Build history of the part. All positions in model axes, mm. A direction names the side the tool comes from. Coordinates: 2 decimals unless noted, no trailing zeros. Loops run counter-clockwise (first coordinate to the right, second up) from the corner with the lowest first, then second, coordinate; pieces in that order, holes last.
Item 1: Cut at D-D (x = 5). List the corners of the cut face in (y, z).
Item 2: Flat gauge pins, fed straight in: pin 1 (0.8 mm diameter, centred on x = 20, y = -9, fed in from -Z); pin 2 (0.6 mm diameter, centred on y = -9, z = 4, fed in from +X); pin 3 (1 mm diameter, centred on y = -7.5, z = 0, fed in from +X). Where does each tip first touch, or does it go through?
Item 3: Cut at A-A (x = 9). List the corners of the cut face in (y, z), and give its area (3 significant figures).
Item 4: Cut at B-B (z = 1.75). List the corners of the cut face in (x, y).
Item 5: 3-axis set-ups, long thin cutter, end or side, ignore diameter. For faces 1 (the face through (10, -8, 0)), 2 (the face through (3.01, -8.76, -3.47)): which of +Z, -Z, +X, -X, +Y, -Y reach the whole face in a straight line?
Item 6: Cut at C-C (y = -6.7). List the corners of the cut face in (x, z), and give its area (3 significant figures).
Item 7: Drill centre lines: line 1 along Y through (x, z) = (25, 0.5); line 2 along X through (y, z) = (-7.3, -0.5). Where is each one in solid material? Low to high.
Item 8: Mould opens along X. For faces 3 (the face through (16, -9.14, 0)), 4 (the face through (3.01, -8.77, 3.54)), 5 (the face through (25, -8, 0)) say: released by +X, released by -X, zero draft, split by the parting line, or undercut.
from build123d import *

# Parameters (mm, degrees)
F0_W      = 0.75
F0_H      = 6
F1_DEPTH  = 33
F2_R      = 1
F3_DEPTH  = 2
F4_R      = 1
F5_W      = 2
F5_H      = 0.75
F6_DEPTH  = 1
F7_SIZE2  = 1.99999
F7_SIZE   = 0.99999
F8_W      = 2
F8_H      = 0.75
F9_DEPTH  = 1
F10_SIZE2 = 1.99999
F10_SIZE  = 0.99999
F12_DEPTH = 25


# Not quite as in the source:
# - a fillet or chamfer is up to 0.001 mm smaller than in the source, because OpenCascade refuses the exact size


with BuildPart() as f1:
    # F0 (on Right) → F1 (new body)
    with BuildSketch(Plane.YZ):
        with Locations((-8.76496256, 0.0332817435)):
            Rectangle(F0_W, F0_H)
    extrude(amount=F1_DEPTH)

    # F2 (on face) → F3 (join)
    with BuildSketch(Plane(origin=(0, -8.38996256, 0), x_dir=(-1, 0, 0), z_dir=(0, 1, 0))):
        with Locations((-9, 0.0332817435)):
            Circle(F2_R)
        with Locations((-24, 0.0332817435)):
            Circle(F2_R)
    extrude(amount=F3_DEPTH)

    # F4
    f4_edges = [f1.edges().sort_by_distance(p)[0] for p in [
        (10, -6.389963, 0.033282),
        (25, -6.389963, 0.033282),
    ]]
    fillet(f4_edges, radius=F4_R)

    # F5 (on face) → F6 (join)
    with BuildSketch(Plane.XY.offset(3.0332817435)):
        with Locations((3, -8.76496256)):
            Rectangle(F5_W, F5_H)
    extrude(amount=F6_DEPTH)

    # F7 (size 1 and 2 in the source; OpenCascade refuses exactly that, so slightly less here)
    f7_edges = [f1.edges().sort_by_distance(p)[0] for p in [
        (2, -8.764963, 4.033282),
    ]]
    f7_side = f1.faces().sort_by_distance((2, -8.764963, 3.533282))[0]
    chamfer(f7_edges, length=F7_SIZE, length2=F7_SIZE2, reference=f7_side)

    # F8 (on face) → F9 (join)
    with BuildSketch(Plane(origin=(0, 0, -2.9667182565), x_dir=(1, 0, 0), z_dir=(0, 0, -1))):
        with Locations((3, 8.76496256)):
            Rectangle(F8_W, F8_H)
    extrude(amount=F9_DEPTH)

    # F10 (size 1 and 2 in the source; OpenCascade refuses exactly that, so slightly less here)
    f10_edges = [f1.edges().sort_by_distance(p)[0] for p in [
        (2, -8.764963, -3.966718),
    ]]
    f10_side = f1.faces().sort_by_distance((2, -8.764963, -3.466718))[0]
    chamfer(f10_edges, length=F10_SIZE, length2=F10_SIZE2, reference=f10_side)

    # F11 (on face) → F12 (cut)
    with BuildSketch(Plane(origin=(0, -8.38996256, 0), x_dir=(-1, 0, 0), z_dir=(0, 1, 0))):
        Polygon((-3, 3.0332817435), (-4, 3.5332817435), (-4, 3.0332817435), align=None)
        Polygon((-3, -2.9667182565), (-4, -2.9667182565), (-4, -3.4667182565), align=None)
    extrude(amount=-F12_DEPTH, mode=Mode.SUBTRACT)


solid = f1.part
Filled sheet:
1. outline: (-9.14, -2.97) - (-8.39, -2.97) - (-8.39, 3.03) - (-9.14, 3.03) - close
2. pin 1: stops at z = -2.97
2. pin 2: stops at x = 4
2. pin 3: stops at x = 25
3. outline: (-9.14, -2.97) - (-8.39, -2.97) - (-8.39, -0.97) - (-7.39, -0.97) arc R1 ccw to (-7.39, 1.03) - (-8.39, 1.03) - (-8.39, 3.03) - (-9.14, 3.03) - close
3. area: 8.07 mm2
4. outline: (0, -9.14) - (33, -9.14) - (33, -8.39) - (0, -8.39) - close
5. face 1: +Y
5. face 2: -Z, -X, +Y, -Y
6. outline: circle Ø1.45 at (9, 0.03); circle Ø1.45 at (24, 0.03)
6. area: 3.29 mm2
7. line 1: y = -9.14 to -8.39
7. line 2: x = 8.16 to 9.84, 23.16 to 24.84
8. face 3: zero draft
8. face 4: released by -X
8. face 5: undercut
